The figure shows three views and two pictorial views of one solid part (mm, origin at its lowest corner). Answer the questions. A direction names the side the tool comes from. Give positions to 0.01 mm unless a question says otherwise; leave off trailing zeros. Write each loop counter-clockwise with the first axis right and the second up, starting at its lowest first coordinate (ties: lowest second). Pieces come first, ordered by that corner, then holes. Notation, with made-up numbers: (81.5, 89) -> (88.5, 89) arc R6 ccw to (88.5, 96) -> close; hole circle Ø3 at (23, 64.25). An arc over 180 degrees is marked (long way). Use a Markdown table: item, result.
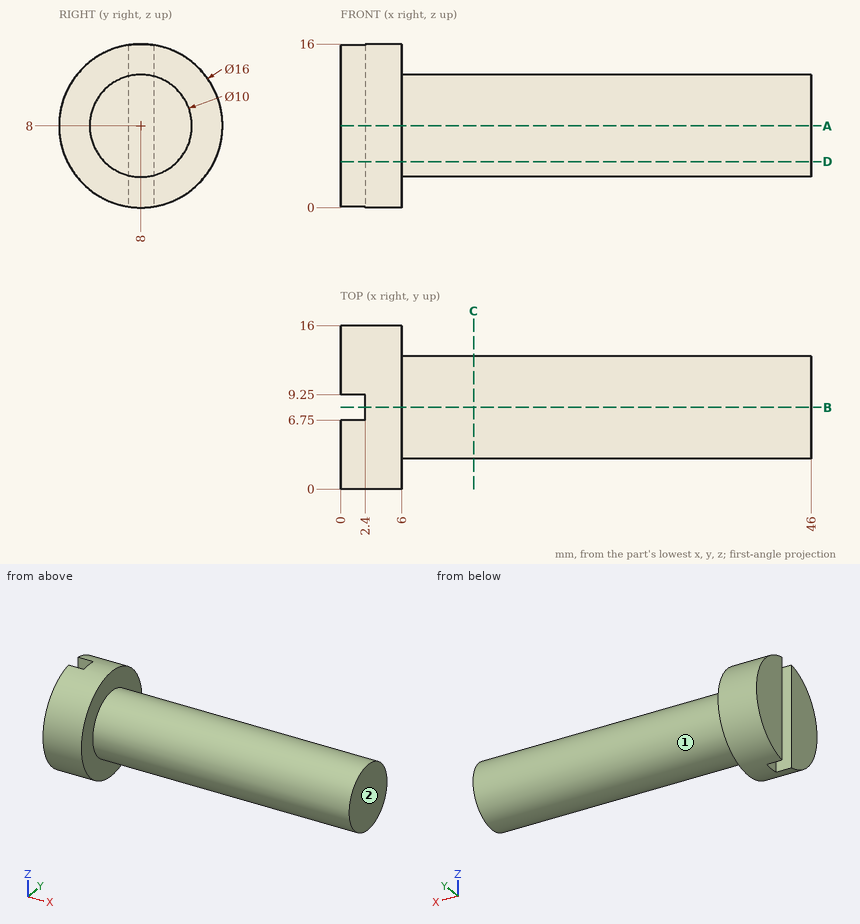
Item 1: Each of these flat-tipped pins is pushed along its axis until it touches: P1, Ø1.2, axis at x = 1.5, z = 4.5, coming from the -Y side; P2, Ø2.5, axis at x = 1.5, z = 11.5, coming from the +Y side; P3, Ø1.2, axis at y = 8, z = 6.5, coming from the -X side. Where does it stop, or does it pass through?
Return value:
| item | result |
|---|---|
| P1 | y = 0.54 |
| P2 | y = 15.68 |
| P3 | x = 2.4 |
Item 2: Straight lines are drawn through the part: line 1 along X through (y, z) = (3.75, 13); line 2 along X through (y, z) = (9, 6.25); line 3 along Y through (x, z) = (2, 11.5). For each, find the intervals that lie inside material, in ascending order. Write a range as [from, to].
Return value:
| item | result |
|---|---|
| line 1 | [0, 6] |
| line 2 | [2.4, 46] |
| line 3 | [0.81, 6.75], [9.25, 15.19] |
Item 3: A cutting plane is placed at D-D (z = 4.5). Give the vertices of the cut face in (x, y), then the cut area to 3 significant figures.
Return value:
| item | result |
|---|---|
| outline | (0, 0.81) -> (6, 0.81) -> (6, 4.43) -> (46, 4.43) -> (46, 11.57) -> (6, 11.57) -> (6, 15.19) -> (0, 15.19) -> (0, 9.25) -> (2.4, 9.25) -> (2.4, 6.75) -> (0, 6.75) -> close |
| area | 366 mm^2 |
Item 4: A cutting plane is placed at A-A (z = 8). Give the vertices of the cut face in (x, y), then the cut area to 3 significant figures.
Return value:
| item | result |
|---|---|
| outline | (0, 0) -> (6, 0) -> (6, 3) -> (46, 3) -> (46, 13) -> (6, 13) -> (6, 16) -> (0, 16) -> (0, 9.25) -> (2.4, 9.25) -> (2.4, 6.75) -> (0, 6.75) -> close |
| area | 490 mm^2 |
Item 5: A cutting plane is placed at B-B (y = 8). Give the vertices of the cut face in (x, z), then the cut area to 3 significant figures.
Return value:
| item | result |
|---|---|
| outline | (2.4, 0) -> (6, 0) -> (6, 3) -> (46, 3) -> (46, 13) -> (6, 13) -> (6, 16) -> (2.4, 16) -> close |
| area | 458 mm^2 |
Item 6: A cutting plane is placed at C-C (x = 13). Give the vertices of the cut face in (y, z), then the cut area to 3 significant figures.
Return value:
| item | result |
|---|---|
| outline | circle Ø10 at (8, 8) |
| area | 78.5 mm^2 |
Item 7: A tool of negligible diameter and unlimited length cuts with its end or side. For the marked faces 1 and 2, from which of +Z, -Z, +X, -X, +Y, -Y can it reach the whole face along a straight path? Write none if from no direction.
Return value:
| item | result |
|---|---|
| face 1 | +X |
| face 2 | +Z, -Z, +X, +Y, -Y |
